from build123d import *

# Parameters (mm, degrees)
F0_W     = 90
F0_H     = 90
F0_R     = 5
F1_DEPTH = 90
F2_R     = 5
F3_W     = 80
F3_H     = 80
F4_DEPTH = 85
F5_W     = 50
F5_H     = 6
F6_DEPTH = 25
F7_W     = 50
F7_H     = 6
F8_DEPTH = 25


with BuildPart() as f1:
    # F0 (on Top) → F1 (new body)
    with BuildSketch(Plane.XY):
        with Locations((45, 45)):
            Rectangle(F0_W, F0_H)
        with Locations((16.019238, 31.732051)):
            Circle(F0_R, mode=Mode.SUBTRACT)
        with Locations((67.980762, 28.267949)):
            Circle(F0_R, mode=Mode.SUBTRACT)
        with Locations((45, 75)):
            Circle(F0_R, mode=Mode.SUBTRACT)
    extrude(amount=F1_DEPTH)

    # F2
    f2_edges = [f1.edges().sort_by_distance(p)[0] for p in [
        (90, 0, 45),
        (90, 90, 45),
        (0, 0, 45),
        (0, 90, 45),
    ]]
    fillet(f2_edges, radius=F2_R)

    # F3 (on face) → F4 (cut)
    with BuildSketch(Plane.XY.offset(90)):
        with Locations((45, 45)):
            Rectangle(F3_W, F3_H)
    extrude(amount=-F4_DEPTH, mode=Mode.SUBTRACT)

    # F5 (on face) → F6 (join)
    with BuildSketch(Plane.XZ):
        with Locations((45, 87)):
            Rectangle(F5_W, F5_H)
    extrude(amount=F6_DEPTH)

    # F7 (on face) → F8 (join)
    with BuildSketch(Plane(origin=(0, 0, 84), x_dir=(1, 0, 0), z_dir=(0, 0, -1))):
        with Locations((45, 22)):
            Rectangle(F7_W, F7_H)
    extrude(amount=F8_DEPTH)


solid = f1.part
Verification items for the finished model (mm, model axes). A direction names the side the tool comes from. Round coordinates to 2 decimals unless told otherwise and drop trailing zeros. Order: outer loops, then holes, each group sorted by start corner. A loop starts at its lowest first (then second) coordinate and runs counter-clockwise, first axis right, second up. Notation, with made-up numbers: (-8, -22.75) -> (16, -22.75) arc R14 ccw to (16, -12.75) -> close; hole circle Ø9 at (61.5, 88.5). An arc over 180 degrees is marked (long way). Put each result on its own line as item: value.
1) Mould release check, pull along Y, two halves, no side actions. Record for faces 5 (the flat face through (44, 85, 48)), 6 (the flat face through (45, -25, 75)), 7 (the cylindrical face through (20.8, 33.2, 2.5)), 8 (the flat face through (44, 90, 44)): +Y half, -Y half, draft (parallel to the pull), parting line (faces both ways), or undercut.
Final values:
face 5: undercut
face 6: -Y half
face 7: undercut
face 8: +Y half
2) Depth check by flat-ended pin: pin 1 (13 mm diameter, centred on x = 67.98, y = 28.27, fed in from +Z); pin 2 (6 mm diameter, centred on x = 16.02, y = 31.73, fed in from -Z) (1 decimal); pin 3 (5 mm diameter, centred on x = 54, y = -23, fed in from -Z); pin 4 (12 mm diameter, centred on x = 53, z = 27.5, fed in from -Y). Enter the tip coordinate at first touch or a pass-through.
Final values:
pin 1: stops at z = 5
pin 2: passes through
pin 3: stops at z = 59
pin 4: stops at y = 0
3) Section check A-A (z = 80.5). Record the cut outline in (x, y).
Final values:
outline: (0, 5) arc R5 ccw to (5, 0) -> (85, 0) arc R5 ccw to (90, 5) -> (90, 85) arc R5 ccw to (85, 90) -> (5, 90) arc R5 ccw to (0, 85) -> close; (20, -25) -> (70, -25) -> (70, -19) -> (20, -19) -> close; hole (5, 5) -> (85, 5) -> (85, 85) -> (5, 85) -> close
4) Section check C-C (y = 75). Record the cut outline in (x, z).
Final values:
outline: (0, 0) -> (40, 0) -> (40, 5) -> (5, 5) -> (5, 90) -> (0, 90) -> close; (50, 0) -> (90, 0) -> (90, 90) -> (85, 90) -> (85, 5) -> (50, 5) -> close
5) Section check D-D (x = 30). Record the cut outline in (y, z), then the cut area to 3 significant figures.
Final values:
outline: (-25, 59) -> (-19, 59) -> (-19, 84) -> (0, 84) -> (0, 0) -> (90, 0) -> (90, 90) -> (85, 90) -> (85, 5) -> (5, 5) -> (5, 90) -> (-25, 90) -> close
area: 1,600 mm^2
6) Set-up check for faces 1 (the flat face through (45, -9, 84)), 2 (the flat face through (44, 46, 5)), 3 (the flat face through (45, -22, 59)), 4 (the flat face through (70, -21, 82)): record each of +Z, -Z, +X, -X, +Y, -Y from which the full face is reachable in a straight line by a thin tool's end or side.
Final values:
face 1: -Z, +X, -X
face 2: +Z
face 3: -Z, +X, -X, -Y
face 4: +Z, -Z, +X, -Y
7) Section check B-B (x = 45). Record the cut outline in (y, z).
Final values:
outline: (-25, 59) -> (-19, 59) -> (-19, 84) -> (0, 84) -> (0, 0) -> (70, 0) -> (70, 5) -> (5, 5) -> (5, 90) -> (-25, 90) -> close; (80, 0) -> (90, 0) -> (90, 90) -> (85, 90) -> (85, 5) -> (80, 5) -> close
8) Material ranges on line 1 (Y direction, x = 58, z = 60); line 2 (X direction, y = 75, z = 3.5); line 3 (X direction, y = 37, z = 27.5), recorded low to high.
Final values:
line 1: y = -25 to -19, 0 to 5, 85 to 90
line 2: x = 0 to 40, 50 to 90
line 3: x = 0 to 5, 85 to 90
